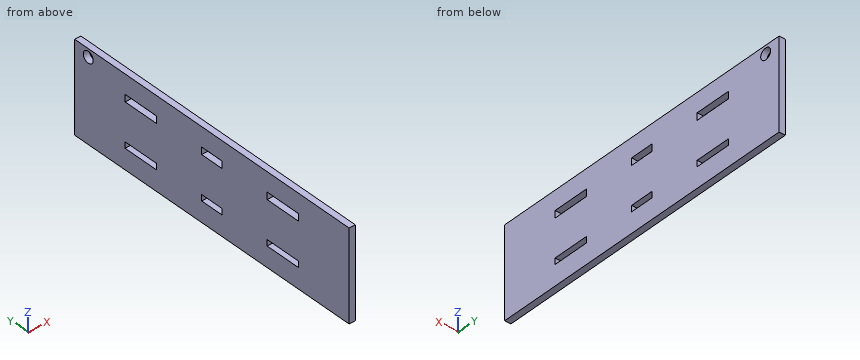
```python
from build123d import *

# Parameters (mm, degrees)
SKETCH1_W           = 304.8
SKETCH1_H           = 88.9
SKETCH1_R           = 5.5
SKETCH1_W_2         = 35
SKETCH1_H_2         = 6
SKETCH1_W_3         = 22.8
SKETCH1_H_3         = 7
BOSS_EXTRUDE1_DEPTH = 6


with BuildPart() as part:
    # Sketch1 → Boss-Extrude1 (new body)
    with BuildSketch(Plane.YZ):
        with Locations((102.640236686, 12.152975526)):
            Rectangle(SKETCH1_W, SKETCH1_H)
        with Locations(Location((240.040236686, 48.602975526, 0), (0, 0, 270))):
            Circle(SKETCH1_R, mode=Mode.SUBTRACT)
        with Locations((23.740236686, -9.297024474)):
            Rectangle(SKETCH1_W_2, SKETCH1_H_2, mode=Mode.SUBTRACT)
        with Locations((102.640236686, -9.297024474)):
            Rectangle(SKETCH1_W_3, SKETCH1_H_2, mode=Mode.SUBTRACT)
        with Locations((181.540236686, -9.297024474)):
            Rectangle(SKETCH1_W_2, SKETCH1_H_2, mode=Mode.SUBTRACT)
        with Locations((23.740236686, 34.202975526)):
            Rectangle(SKETCH1_W_2, SKETCH1_H_3, mode=Mode.SUBTRACT)
        with Locations((102.640236686, 34.202975526)):
            Rectangle(SKETCH1_W_3, SKETCH1_H_3, mode=Mode.SUBTRACT)
        with Locations((181.540236686, 34.202975526)):
            Rectangle(SKETCH1_W_2, SKETCH1_H_3, mode=Mode.SUBTRACT)
    extrude(amount=BOSS_EXTRUDE1_DEPTH)


solid = part.part
```
The listing builds one solid part. Answer for the finished solid, in the listing's coordinates (mm). Round coordinates to 2 decimals unless told otherwise and drop trailing zeros. Loops run counter-clockwise (first coordinate to the right, second up) from the corner with the lowest first, then second, coordinate; pieces in that order, holes last.
Q1. Section B-B, the plane z = 35 is taken. Determine the outline of the cut face in (x, y).
Q2. Section A-A, the plane y = 107 is taken. Determine the outline of the cut face in (x, z).
Q3. Section C-C, the plane x = 0.95 is taken. Count the separate pieces of the cut face and the enclosed holes in it, then the cut area to 3 significant figures.
Q4. Find the intervals of material crossed by line 1 (Y direction, x = 1.5, z = 36.5); line 2 (Z direction, x = 3.25, y = 100.5); line 3 (Z direction, x = 4, y = 238), in increasing order.
Completed:
1. outline: (0, -49.76) - (6, -49.76) - (6, 6.24) - (0, 6.24) - close; (0, 41.24) - (6, 41.24) - (6, 91.24) - (0, 91.24) - close; (0, 114.04) - (6, 114.04) - (6, 164.04) - (0, 164.04) - close; (0, 199.04) - (6, 199.04) - (6, 255.04) - (0, 255.04) - close
2. outline: (0, -32.3) - (6, -32.3) - (6, -12.3) - (0, -12.3) - close; (0, -6.3) - (6, -6.3) - (6, 30.7) - (0, 30.7) - close; (0, 37.7) - (6, 37.7) - (6, 56.6) - (0, 56.6) - close
3. separate pieces: 1
3. enclosed holes: 7
3. area: 25,800 mm2
4. line 1: y = -49.76 to 6.24, 41.24 to 91.24, 114.04 to 164.04, 199.04 to 255.04
4. line 2: z = -32.3 to -12.3, -6.3 to 30.7, 37.7 to 56.6
4. line 3: z = -32.3 to 43.5, 53.71 to 56.6
